Autodesk Inventor part; units mm, degrees
ref_plane "YZ Plane" through (0, 0, 0) normal (1, 0, 0) x (0, 1, 0)
ref_plane "XZ Plane" through (0, 0, 0) normal (0, 1, 0) x (-1, 0, 0)
ref_plane "XY Plane" through (0, 0, 0) normal (0, 0, 1) x (1, 0, 0)
sketch "Sketch4" plane through (0, 0, 0) normal (0, 0, 1) x (1, 0, 0)
  line L0 (0, 0) -> (-25, 0)
  line L1 (-25, 0) -> (-25, 2.5)
  line L2 (-25, 2.5) -> (-10, 2.5)
  line L3 (-10, 2.5) -> (-10, 40)
  line L4 (-10, 40) -> (-7.5, 40)
  line L5 (-7.5, 40) -> (-7.5, 15)
  line L6 (-7.5, 15) -> (0, 15)
  line L7 (0, 15) -> (0, 0)
  line L8 (0, 0) -> (25, 0)
  line L9 (25, 0) -> (25, 2.5)
  line L10 (25, 2.5) -> (10, 2.5)
  line L11 (10, 2.5) -> (10, 40)
  line L12 (10, 40) -> (7.5, 40)
  line L13 (7.5, 40) -> (7.5, 15)
  line L14 (7.5, 15) -> (0, 15)
  dimension "d43" = 25
  dimension "d44" = 2.5
  dimension "d45" = 15
  dimension "d46" = 37.5
  dimension "d47" = 2.5
  dimension "d48" = 25
extrude "Extrusion3" add sketch "Sketch4" along normal blind 10
fillet "Fillet6" radius 5 4 edges at (8.75, 40, 10) (8.75, 40, 0) (-8.75, 40, 0) (-8.75, 40, 10)
chamfer "Chamfer1" distance 0.5 angle 45 11 edges at (17.5, 2.5, 0) (25, 2.5, 5) (17.5, 2.5, 10) (-17.5, 2.5, 0) (-25, 2.5, 5) (-17.5, 2.5, 10) (-12.5, 0, 0) (-25, 0, 5) (-12.5, 0, 10) (25, 0, 5) (25, 1.25, 0)
sketch "Sketch5" plane through (-24.5, 2.5, 0.5) normal (0, 1, 0) x (1, 0, 0)
  line L0 (0, -9) -> (0, 0)
  line L1 (0, 0) -> (14.5, 0)
  point P0 (24.5, 0.5)
  point P1 (9.5, -4)
  dimension "d57" = 9.5
  dimension "d58" = 4
hole "Hole2" at (-15, 2.5, 4.5) direction (0, -1, 0) diameter 4 end through all
thread "Thread3"
mirror "Mirror1" about plane through (0, 0, 0) normal (1, 0, 0) of "Hole2"
sketch "Sketch6" plane through (10, 35, 5) normal (1, 0, 0) x (0, 0, -1)
  arc A0 (5, 0) -> (-5, 0) centre (0, 0) ccw
  point P0 (5, -35)
hole "Hole3" at (10, 35, 5) direction (-1, 0, 0) diameter 8 end through all
chamfer "Chamfer2" distance 4 angle 45 1 edges at (0, 15, 10)
chamfer "Chamfer3" distance 4 angle 45 1 edges at (0, 15, 0)
properties part number "Bearing Block"
Part model, mm, in its own coordinate system. A direction names the side the tool comes from. Coordinates: 2 decimals unless noted, no trailing zeros. Write each loop counter-clockwise with the first axis right and the second up, starting at its lowest first coordinate (ties: lowest second). Pieces come first, ordered by that corner, then holes. Notation, with made-up numbers: M -2,56.5 L 16,56.5 A29 ccw 16,93.5 Z; hole C 22.5,6 d3. An arc over 180 degrees is marked long. Return JSON: item names as keys, results as strings.
1. Saw through at D-D, the plane x = -5.5. Write the cut outline in (y, z), then the cut area to 3 significant figures.
Determined:
{"outline": "M 0,0.5 L 0.5,0 L 11,0 L 15,4 L 15,6 L 11,10 L 0.5,10 L 0,9.5 Z", "area": "134 mm²"}
2. Saw through at C-C, the plane z = 8. Write the cut outline in (x, y), then the cut area to 3 significant figures.
Determined:
{"outline": "M -25,0.5 L -24.5,0 L 24.5,0 L 25,0.5 L 25,2 L 24.5,2.5 L 10,2.5 L 10,32.35 L 7.5,32.35 L 7.5,13 L -7.5,13 L -7.5,32.35 L -10,32.35 L -10,2.5 L -24.5,2.5 L -25,2 Z; M -10,37.65 L -7.5,37.65 L -7.5,39 L -10,39 Z; M 7.5,37.65 L 10,37.65 L 10,39 L 7.5,39 Z", "area": "438 mm²"}
3. Pull direction X, two halves, no side cores. Call faces 1 (the face through (10, 17, 5)), 2 (the face through (-7.5, 22, 5)), 3 (the face through (-17.4, 2.5, 4.9)): pulls with the +X half, pulls with the -X half, needs draft (parallel to the pull), parting line crosses it, or undercut.
Determined:
{"face 1": "pulls with the +X half", "face 2": "undercut", "face 3": "needs draft"}
4. 3-axis set-ups, long thin cutter, end or side, ignore diameter. For faces 4 (the face through (17.4, 2.5, 4.9)), 5 (the face through (0, 13, 2)), 6 (the face through (0, 15, 5)): which of +Z, -Z, +X, -X, +Y, -Y reach the whole face in a straight line?
Determined:
{"face 4": "+Z, -Z, +X, +Y", "face 5": "-Z, +Y", "face 6": "+Z, -Z, +Y"}
5. Saw through at A-A, the plane y = 28.5. Write the cut outline in (x, z), then the cut area to 3 significant figures.
Determined:
{"outline": "M -10,0 L -7.5,0 L -7.5,10 L -10,10 Z; M 7.5,0 L 10,0 L 10,10 L 7.5,10 Z", "area": "50.0 mm²"}
6. Probe L1, parallel to X at y = 1.45, z = 4.5; L2, parallel to X at y = 30, z = 5.75; L3, parallel to Y at x = -9.4, z = 5. List the from-to ranges inside material, lowest first.
Determined:
{"L1": "-25 to -17, -13 to 13, 17 to 25", "L2": "-10 to -7.5, 7.5 to 10", "L3": "0 to 31, 39 to 40"}
7. Saw through at B-B, the plane x = 15. Write the cut outline in (y, z).
Determined:
{"outline": "M 0,0.5 L 0.5,0 L 2,0 L 2.5,0.5 L 2.5,2.5 L 0,2.5 Z; M 0,6.5 L 2.5,6.5 L 2.5,9.5 L 2,10 L 0.5,10 L 0,9.5 Z"}
8. Flat gauge pins, fed straight in: pin 1 Ø2 at (y, z) = (9, 6.5) entering from -X; pin 2 Ø1.6 at (x, z) = (-3, 5.5) entering from +Y; pin 3 Ø2.5 at (x, z) = (18, 4) entering from +Y. Where does each tip first touch, or does it go through?
Determined:
{"pin 1": "x = -10", "pin 2": "y = 15", "pin 3": "y = 2.5"}
